The listing builds one solid part. Answer for the finished solid, in the listing's coordinates (mm). Give positions to 0.01 mm unless a question says otherwise; leave off trailing zeros. Order: outer loops, then holes, each group sorted by start corner. A loop starts at its lowest first (then second) coordinate and runs counter-clockwise, first axis right, second up.
```python
from build123d import *

# Parameters (mm, degrees)
SKETCH1_W           = 16.86
SKETCH1_H           = 25.88
BOSS_EXTRUDE1_DEPTH = 1.5
CUT_EXTRUDE1_REACH  = 3.5
SKETCH2_R           = 1.5
CUT_EXTRUDE2_REACH  = 3.5
SKETCH3_R           = 0.8


with BuildPart() as part:
    # Sketch1 → Boss-Extrude1 (new body)
    with BuildSketch(Plane(origin=(0, 0, 0), x_dir=(1, 0, 0), z_dir=(0, 1, 0))):
        with Locations((8.43, 12.94)):
            Rectangle(SKETCH1_W, SKETCH1_H)
    extrude(amount=BOSS_EXTRUDE1_DEPTH)

    # Sketch2 → Cut-Extrude1 (cut, up to next)
    with BuildSketch(Plane(origin=(0, 1.5, 0), x_dir=(1, 0, 0), z_dir=(0, 1, 0)), mode=Mode.PRIVATE) as cut_extrude1_sk1:
        with Locations((14.26, 23.24)):
            Circle(SKETCH2_R)
    cut_extrude1_tool1 = extrude(cut_extrude1_sk1.sketch, amount=-CUT_EXTRUDE1_REACH, mode=Mode.PRIVATE) & part.part
    add(cut_extrude1_tool1.solids().sort_by_distance((14.26, 1.5, -23.24))[0], mode=Mode.SUBTRACT)
    # Sketch2 → Cut-Extrude1 (cut, up to next)
    with BuildSketch(Plane(origin=(0, 1.5, 0), x_dir=(1, 0, 0), z_dir=(0, 1, 0)), mode=Mode.PRIVATE) as cut_extrude1_sk2:
        with Locations((14.26, 2.64)):
            Circle(SKETCH2_R)
    cut_extrude1_tool2 = extrude(cut_extrude1_sk2.sketch, amount=-CUT_EXTRUDE1_REACH, mode=Mode.PRIVATE) & part.part
    add(cut_extrude1_tool2.solids().sort_by_distance((14.26, 1.5, -2.64))[0], mode=Mode.SUBTRACT)

    # Sketch3 → Cut-Extrude2 (cut, up to next)
    with BuildSketch(Plane(origin=(0, 1.5, 0), x_dir=(1, 0, 0), z_dir=(0, 1, 0)), mode=Mode.PRIVATE) as cut_extrude2_sk1:
        with Locations((1.58, 24.32)):
            Circle(SKETCH3_R)
    cut_extrude2_tool1 = extrude(cut_extrude2_sk1.sketch, amount=-CUT_EXTRUDE2_REACH, mode=Mode.PRIVATE) & part.part
    add(cut_extrude2_tool1.solids().sort_by_distance((1.58, 1.5, -24.32))[0], mode=Mode.SUBTRACT)
    # Sketch3 → Cut-Extrude2 (cut, up to next)
    with BuildSketch(Plane(origin=(0, 1.5, 0), x_dir=(1, 0, 0), z_dir=(0, 1, 0)), mode=Mode.PRIVATE) as cut_extrude2_sk2:
        with Locations((1.58, 21.78)):
            Circle(SKETCH3_R)
    cut_extrude2_tool2 = extrude(cut_extrude2_sk2.sketch, amount=-CUT_EXTRUDE2_REACH, mode=Mode.PRIVATE) & part.part
    add(cut_extrude2_tool2.solids().sort_by_distance((1.58, 1.5, -21.78))[0], mode=Mode.SUBTRACT)
    # Sketch3 → Cut-Extrude2 (cut, up to next)
    with BuildSketch(Plane(origin=(0, 1.5, 0), x_dir=(1, 0, 0), z_dir=(0, 1, 0)), mode=Mode.PRIVATE) as cut_extrude2_sk3:
        with Locations((1.58, 19.24)):
            Circle(SKETCH3_R)
    cut_extrude2_tool3 = extrude(cut_extrude2_sk3.sketch, amount=-CUT_EXTRUDE2_REACH, mode=Mode.PRIVATE) & part.part
    add(cut_extrude2_tool3.solids().sort_by_distance((1.58, 1.5, -19.24))[0], mode=Mode.SUBTRACT)
    # Sketch3 → Cut-Extrude2 (cut, up to next)
    with BuildSketch(Plane(origin=(0, 1.5, 0), x_dir=(1, 0, 0), z_dir=(0, 1, 0)), mode=Mode.PRIVATE) as cut_extrude2_sk4:
        with Locations((1.58, 16.7)):
            Circle(SKETCH3_R)
    cut_extrude2_tool4 = extrude(cut_extrude2_sk4.sketch, amount=-CUT_EXTRUDE2_REACH, mode=Mode.PRIVATE) & part.part
    add(cut_extrude2_tool4.solids().sort_by_distance((1.58, 1.5, -16.7))[0], mode=Mode.SUBTRACT)
    # Sketch3 → Cut-Extrude2 (cut, up to next)
    with BuildSketch(Plane(origin=(0, 1.5, 0), x_dir=(1, 0, 0), z_dir=(0, 1, 0)), mode=Mode.PRIVATE) as cut_extrude2_sk5:
        with Locations((1.58, 14.16)):
            Circle(SKETCH3_R)
    cut_extrude2_tool5 = extrude(cut_extrude2_sk5.sketch, amount=-CUT_EXTRUDE2_REACH, mode=Mode.PRIVATE) & part.part
    add(cut_extrude2_tool5.solids().sort_by_distance((1.58, 1.5, -14.16))[0], mode=Mode.SUBTRACT)
    # Sketch3 → Cut-Extrude2 (cut, up to next)
    with BuildSketch(Plane(origin=(0, 1.5, 0), x_dir=(1, 0, 0), z_dir=(0, 1, 0)), mode=Mode.PRIVATE) as cut_extrude2_sk6:
        with Locations((1.58, 11.62)):
            Circle(SKETCH3_R)
    cut_extrude2_tool6 = extrude(cut_extrude2_sk6.sketch, amount=-CUT_EXTRUDE2_REACH, mode=Mode.PRIVATE) & part.part
    add(cut_extrude2_tool6.solids().sort_by_distance((1.58, 1.5, -11.62))[0], mode=Mode.SUBTRACT)
    # Sketch3 → Cut-Extrude2 (cut, up to next)
    with BuildSketch(Plane(origin=(0, 1.5, 0), x_dir=(1, 0, 0), z_dir=(0, 1, 0)), mode=Mode.PRIVATE) as cut_extrude2_sk7:
        with Locations((1.58, 9.08)):
            Circle(SKETCH3_R)
    cut_extrude2_tool7 = extrude(cut_extrude2_sk7.sketch, amount=-CUT_EXTRUDE2_REACH, mode=Mode.PRIVATE) & part.part
    add(cut_extrude2_tool7.solids().sort_by_distance((1.58, 1.5, -9.08))[0], mode=Mode.SUBTRACT)
    # Sketch3 → Cut-Extrude2 (cut, up to next)
    with BuildSketch(Plane(origin=(0, 1.5, 0), x_dir=(1, 0, 0), z_dir=(0, 1, 0)), mode=Mode.PRIVATE) as cut_extrude2_sk8:
        with Locations((1.58, 6.54)):
            Circle(SKETCH3_R)
    cut_extrude2_tool8 = extrude(cut_extrude2_sk8.sketch, amount=-CUT_EXTRUDE2_REACH, mode=Mode.PRIVATE) & part.part
    add(cut_extrude2_tool8.solids().sort_by_distance((1.58, 1.5, -6.54))[0], mode=Mode.SUBTRACT)
    # Sketch3 → Cut-Extrude2 (cut, up to next)
    with BuildSketch(Plane(origin=(0, 1.5, 0), x_dir=(1, 0, 0), z_dir=(0, 1, 0)), mode=Mode.PRIVATE) as cut_extrude2_sk9:
        with Locations((1.58, 4)):
            Circle(SKETCH3_R)
    cut_extrude2_tool9 = extrude(cut_extrude2_sk9.sketch, amount=-CUT_EXTRUDE2_REACH, mode=Mode.PRIVATE) & part.part
    add(cut_extrude2_tool9.solids().sort_by_distance((1.58, 1.5, -4))[0], mode=Mode.SUBTRACT)
    # Sketch3 → Cut-Extrude2 (cut, up to next)
    with BuildSketch(Plane(origin=(0, 1.5, 0), x_dir=(1, 0, 0), z_dir=(0, 1, 0)), mode=Mode.PRIVATE) as cut_extrude2_sk10:
        with Locations((1.58, 1.46)):
            Circle(SKETCH3_R)
    cut_extrude2_tool10 = extrude(cut_extrude2_sk10.sketch, amount=-CUT_EXTRUDE2_REACH, mode=Mode.PRIVATE) & part.part
    add(cut_extrude2_tool10.solids().sort_by_distance((1.58, 1.5, -1.46))[0], mode=Mode.SUBTRACT)


solid = part.part
```
1) Find section B-B (z = -6.54). Write down the section's boundary in (x, y), then the cut area to 3 significant figures.
Geometry says:
outline: (0, 0) - (0.78, 0) - (0.78, 1.5) - (0, 1.5) - close; (2.38, 0) - (16.86, 0) - (16.86, 1.5) - (2.38, 1.5) - close
area: 22.9 mm2
2) For a pull along X with two mould halves and no side action, classify faces 1 (the flat face through (0, 1, -13)), 2 (the cylindrical face through (1.41, 0.76, -5.76)), 3 (the flat face through (8, 1.5, -13)) as +X half, -X half, draft (parallel to the pull), parting line (faces both ways), or undercut.
Geometry says:
face 1: -X half
face 2: undercut
face 3: draft
3) Find section D-D (z = -24.32). Write down the section's boundary in (x, y).
Geometry says:
outline: (0, 0) - (0.78, 0) - (0.78, 1.5) - (0, 1.5) - close; (2.38, 0) - (13.22, 0) - (13.22, 1.5) - (2.38, 1.5) - close; (15.3, 0) - (16.86, 0) - (16.86, 1.5) - (15.3, 1.5) - close
4) Straight lines are drawn through the part: probe 1 along Z at (x, y) = (14.26, 0.35); probe 2 along X at (y, z) = (0.4, -11.62); probe 3 along Z at (x, y) = (13, 0.5). For each, find the intervals that lie inside material, in ascending order.
Geometry says:
probe 1: z = -25.88 to -24.74, -21.74 to -4.14, -1.14 to 0
probe 2: x = 0 to 0.78, 2.38 to 16.86
probe 3: z = -25.88 to -24.05, -22.43 to -3.45, -1.83 to 0
5) Find section A-A (y = 0.45). Count the separate pieces of the cut face and the enclosed holes in it, then the cut area to 3 significant figures.
Geometry says:
separate pieces: 1
enclosed holes: 12
area: 402 mm2
